```python
from build123d import *

# Parameters (mm, degrees)
F1_DEPTH = 63.5
F0_W     = 25.4
F0_H     = 19.05
F2_DEPTH = 25.4
F3_DEPTH = 7.9375
F5_SIZE  = 6.35


# Not quite as in the source:
# - a feature names something its author has since deleted; it is built from what else it names


with BuildPart() as f1:
    # F0 (on Front) → F1 (new body, symmetric)
    with BuildSketch(Plane.XZ):
        Polygon((-41.275, 9.525), (-41.275, -9.525), (41.275, -9.525), (41.275, 9.525), (22.225, 9.525), align=None)
    extrude(amount=F1_DEPTH, both=True)

    # F0 (on Front) → F2 (join, symmetric)
    with BuildSketch(Plane.XZ):
        with BuildLine():
            Line((22.225, 9.525), (41.275, 9.525))
            Line((41.275, 9.525), (41.275, 27.0002))
            ThreePointArc((41.275, 27.0002), (45.9246798487, 38.2255201513), (57.15, 42.8752))
            Line((57.15, 42.8752), (60.325, 42.8752))
            Line((60.325, 42.8752), (60.325, 61.9252))
            Line((60.325, 61.9252), (57.15, 61.9252))
            ThreePointArc((57.15, 61.9252), (32.4542956671, 51.6959043329), (22.225, 27.0002))
            Line((22.225, 27.0002), (22.225, 9.525))
        make_face()
        with Locations((73.025, 52.4002)):
            Rectangle(F0_W, F0_H)
    extrude(amount=F2_DEPTH, both=True)

    # F0 (on Front) → F3 (join, symmetric)
    with BuildSketch(Plane.XZ):
        with BuildLine():
            add(Edge.make_bspline(
                [(-41.275, 9.525), (-41.0928055644, 45.868396759), (20.8572410047, 62.0456375182), (57.15, 61.9252)],
                knots=[0, 0, 0, 0, 111.5045361635, 111.5045361635, 111.5045361635, 111.5045361635], degree=3))
            Line((-41.275, 9.525), (22.225, 9.525))
            Line((22.225, 9.525), (22.225, 27.0002))
            ThreePointArc((22.225, 27.0002), (32.4542956671, 51.6959043329), (57.15, 61.9252))
        make_face()
    extrude(amount=F3_DEPTH, both=True)

    # F0 (on Front) → F4 (revolve)
    with BuildSketch(Plane.XZ):
        Polygon((85.725, 66.675), (85.725, 61.9252), (85.725, 42.8752), (85.725, 38.1), (111.125, 38.1), (111.125, 66.675), align=None)
    revolve(axis=Axis((85.725, 0, 52.3875), (0, 0, -1)))

    # F5
    f5_edges = [f1.edges().sort_by_distance(p)[0] for p in [
        (41.275, -63.5, 0),
        (-41.275, -63.5, 0),
        (41.275, 63.5, 0),
        (-41.275, 63.5, 0),
    ]]
    chamfer(f5_edges, length=F5_SIZE)


solid = f1.part
```
Here's how the part is built. I have some questions about the finished solid (model axes, mm). A direction names the side the tool comes from. Round coordinates to 2 decimals unless told otherwise and drop trailing zeros. Write each loop counter-clockwise with the first axis right and the second up, starting at its lowest first coordinate (ties: lowest second). Pieces come first, ordered by that corner, then holes.
Q1. Will these pins go through, and if not, where does the flat tip stop? P1, Ø2, axis at x = 9, z = 24.5, coming from the -Y side; P2, Ø12, axis at y = 6, z = 44.5, coming from the -X side; P3, Ø5, axis at x = 34, z = 15, coming from the -Y side; P4, Ø19, axis at y = -14, z = 18.5, coming from the -X side (3 decimals).
Q2. If we mould it in two halves opening along X, with no side actions, what happens to faces 5 (the flat face through (-1, -1, -9.525)), 6 (the flat face through (60, 2, 42.875)), 7 (the cylindrical face through (45.8, -0.4, 38.1)), 8 (the cylindrical face through (32.73, -16.79, 51.97))? For each: +X half, -X half, draft (parallel to the pull), parting line (faces both ways), or undercut.
Q3. If we section it at A-A on z = 1.5: Write out the boundary of the cut face in (x, y) (3 decimals), plus the area to 3 significant figures.
Q4. If we section it at D-D on y = 30: Write out the boundary of the cut face in (x, z) (3 decimals).
Q5. Which directions (+Z, -Z, +X, -X, +Y, -Y) give clear straight access to the entire face, cutting with the end or side of a thin tool? Please do faces 1 (the flat face through (22.225, -17, 18)), 2 (the flat face through (60, -2, 61.925)), 3 (the flat face through (22.225, 17, 18)), 4 (the flat face through (46, 25.4, 42)).
Q6. Please list where these lines run through material, in increasing order: probe 1 along X at (y, z) = (24, 13.5) (3 decimals); probe 2 along Z at (x, y) = (-27, -46) (3 decimals); probe 3 along Y at (x, z) = (-27, 29).
Q7. If we section it at C-C on x = 72: Write out the boundary of the cut face in (y, z) (3 decimals), plus the area to 3 significant figures.
Q8. If we section it at B-B on y = -15.5: Write out the boundary of the cut face in (x, z) (3 decimals).
Answer below:
1. P1: stops at y = -7.94
1. P2: stops at x = -24.79
1. P3: stops at y = -25.4
1. P4: stops at x = -41.275
2. face 5: draft
2. face 6: undercut
2. face 7: undercut
2. face 8: -X half
3. outline: (-41.275, -57.15) - (-34.925, -63.5) - (34.925, -63.5) - (41.275, -57.15) - (41.275, 57.15) - (34.925, 63.5) - (-34.925, 63.5) - (-41.275, 57.15) - close
3. area: 10,400 mm2
4. outline: (-41.275, -9.525) - (41.275, -9.525) - (41.275, 9.525) - (-41.275, 9.525) - close
5. face 1: +Z, -X, -Y
5. face 2: +Z, -X
5. face 3: +Z, -X, +Y
5. face 4: +Z, +X, -X, +Y
6. probe 1: x = 22.225 to 41.275
6. probe 2: z = -9.525 to 9.525
6. probe 3: y = -7.94 to 7.94
7. outline: (-25.4, 42.875) - (-21.373, 42.875) - (-21.373, 38.1) - (21.373, 38.1) - (21.373, 42.875) - (25.4, 42.875) - (25.4, 61.925) - (21.373, 61.925) - (21.373, 66.675) - (-21.373, 66.675) - (-21.373, 61.925) - (-25.4, 61.925) - close
7. area: 1,370 mm2
8. outline: (-41.275, -9.525) - (41.275, -9.525) - (41.275, 27) arc R15.875 cw to (57.15, 42.875) - (65.603, 42.875) - (65.603, 38.1) - (105.847, 38.1) - (105.847, 66.675) - (65.603, 66.675) - (65.603, 61.925) - (57.15, 61.925) arc R34.925 ccw to (22.225, 27) - (22.225, 9.525) - (-41.275, 9.525) - close
